Verification items for the finished model (mm, model axes). Face numbers are marked on the shaded views. A direction names the side the tool comes from. Give positions to 0.01 mm unless a question says otherwise; leave off trailing zeros. Write each loop counter-clockwise with the first axis right and the second up, starting at its lowest first coordinate (ties: lowest second). Pieces come first, ordered by that corner, then holes.
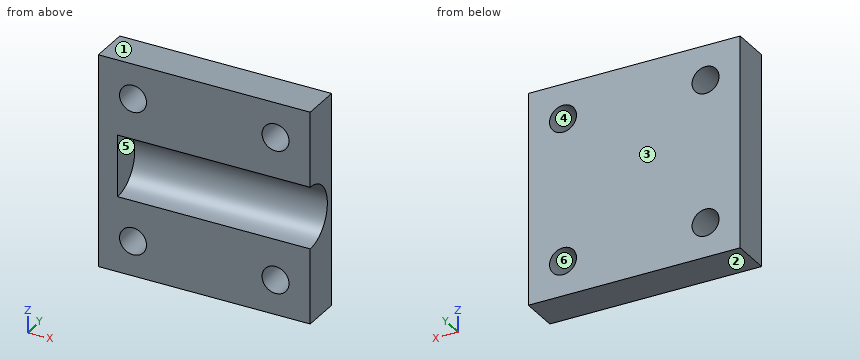
from build123d import *

# Parameters (mm, degrees)
SKETCH1_W           = 55
SKETCH1_H           = 55
BOSS_EXTRUDE1_DEPTH = 10
SKETCH2_R           = 8
CUT_EXTRUDE1_DEPTH  = 50
SKETCH3_R           = 3.5
CUT_EXTRUDE2_DEPTH  = 50


with BuildPart() as part:
    # Sketch1 → Boss-Extrude1 (new body)
    with BuildSketch(Plane(origin=(0, 0, 0), x_dir=(1, 0, 0), z_dir=(0, 1, 0))):
        Rectangle(SKETCH1_W, SKETCH1_H)
    extrude(amount=BOSS_EXTRUDE1_DEPTH)

    # Sketch2 → Cut-Extrude1 (cut)
    with BuildSketch(Plane(origin=(27.5, 0, 0), x_dir=(0, 0, -1), z_dir=(1, 0, 0))):
        Circle(SKETCH2_R)
    extrude(amount=-CUT_EXTRUDE1_DEPTH, mode=Mode.SUBTRACT)

    # Sketch3 → Cut-Extrude2 (cut)
    with BuildSketch(Plane(origin=(0, 10, 0), x_dir=(1, 0, 0), z_dir=(0, 1, 0))):
        with Locations((-18.5, 18.5)):
            Circle(SKETCH3_R)
        with Locations((18.5, 18.5)):
            Circle(SKETCH3_R)
        with Locations((-18.5, -18.5)):
            Circle(SKETCH3_R)
        with Locations((18.5, -18.5)):
            Circle(SKETCH3_R)
    extrude(amount=-CUT_EXTRUDE2_DEPTH, mode=Mode.SUBTRACT)


solid = part.part
Item 1: Sectioned sample at B-B on x = 18.5. Record the cut outline in (y, z).
Answer key:
outline: (0, -27.5) - (10, -27.5) - (10, -22) - (0, -22) - close; (0, -15) - (10, -15) - (10, 15) - (0, 15) - (0, 8) arc R8 cw to (0, -8) - close; (0, 22) - (10, 22) - (10, 27.5) - (0, 27.5) - close
Item 2: Sectioned sample at D-D on z = 17.5. Record the cut outline in (x, y).
Answer key:
outline: (-27.5, 0) - (-21.85, 0) - (-21.85, 10) - (-27.5, 10) - close; (-15.15, 0) - (15.15, 0) - (15.15, 10) - (-15.15, 10) - close; (21.85, 0) - (27.5, 0) - (27.5, 10) - (21.85, 10) - close
Item 3: Sectioned sample at A-A on z = -18.5. Record the cut outline in (x, y), then the cut area to 3 significant figures.
Answer key:
outline: (-27.5, 0) - (-22, 0) - (-22, 10) - (-27.5, 10) - close; (-15, 0) - (15, 0) - (15, 10) - (-15, 10) - close; (22, 0) - (27.5, 0) - (27.5, 10) - (22, 10) - close
area: 410 mm2
Item 4: Scan lines: line 1 along X through (y, z) = (5.5, 18.5); line 2 along Z through (x, y) = (18.5, 2.25); line 3 along Z through (x, y) = (-18.5, 5.5). Record each from-to range of solid material in increasing order.
Answer key:
line 1: x = -27.5 to -22, -15 to 15, 22 to 27.5
line 2: z = -27.5 to -22, -15 to -7.68, 7.68 to 15, 22 to 27.5
line 3: z = -27.5 to -22, -15 to -5.81, 5.81 to 15, 22 to 27.5
Item 5: Sectioned sample at C-C on y = 6.5. Record the cut outline in (x, z).
Answer key:
outline: (-27.5, -27.5) - (27.5, -27.5) - (27.5, -4.66) - (-22.5, -4.66) - (-22.5, 4.66) - (27.5, 4.66) - (27.5, 27.5) - (-27.5, 27.5) - close; hole circle Ø7 at (-18.5, -18.5); hole circle Ø7 at (-18.5, 18.5); hole circle Ø7 at (18.5, -18.5); hole circle Ø7 at (18.5, 18.5)
Item 6: Depth check by flat-ended pin: pin 1 (4 mm diameter, centred on y = 2.5, z = -2.5, fed in from +X). Enter the tip coordinate at first touch or a pass-through.
Answer key:
pin 1: stops at x = -22.5
Item 7: Set-up check for the marked faces 5 and 6: record each of +Z, -Z, +X, -X, +Y, -Y from which the full face is reachable in a straight line by a thin tool's end or side.
Answer key:
face 5: +X, -Y
face 6: +Y, -Y
Item 8: Release check for a two-part mould opening along Z. For the marked faces 1, 2, 3 and 4 record: released by +Z, released by -Z, zero draft, split by the parting line, or undercut.
Answer key:
face 1: released by +Z
face 2: released by -Z
face 3: zero draft
face 4: undercut
